The figure shows three views and two pictorial views of one solid part (mm, origin at its lowest corner). Answer the questions. Round coordinates to 2 decimals unless told otherwise and drop trailing zeros. Order: outer loops, then holes, each group sorted by start corner. A loop starts at its lowest first (then second) coordinate and runs counter-clockwise, first axis right, second up. Notation, with made-up numbers: (-18.5, 71) -> (-12.5, 71) arc R18 cw to (-12.5, 99) -> close; hole circle Ø11 at (59, 30.25). An arc over 180 degrees is marked (long way). One line per item, written item: value. Start each with the question number.
1. Section D-D (x = 7) is taken. Give the vertices of the cut face in (y, z).
2. Flat-ended cylindrical pins translate along their axes: pin 1 Ø1.5 at (y, z) = (1, 1.5) entering from -X; pin 2 Ø1.5 at (y, z) = (1, 55) entering from -X. Find the tip coordinate at first contact, or state that the pin passes through.
3. Consider line 1 (X direction, y = 0.2, z = 60); line 2 (Z direction, x = 29, y = 2.15); line 3 (X direction, y = 2.05, z = 71). Determine where each line is inside the solid, lowest interval first.
4. Section B-B (y = 2.55) is taken. Give the vertices of the cut face in (x, z), then the cut area to 3 significant figures.
5. Section A-A (z = 49.5) is taken. Give the vertices of the cut face in (x, y).
6. Section C-C (x = 21) is taken. Give the vertices of the cut face in (y, z), then the cut area to 3 significant figures.
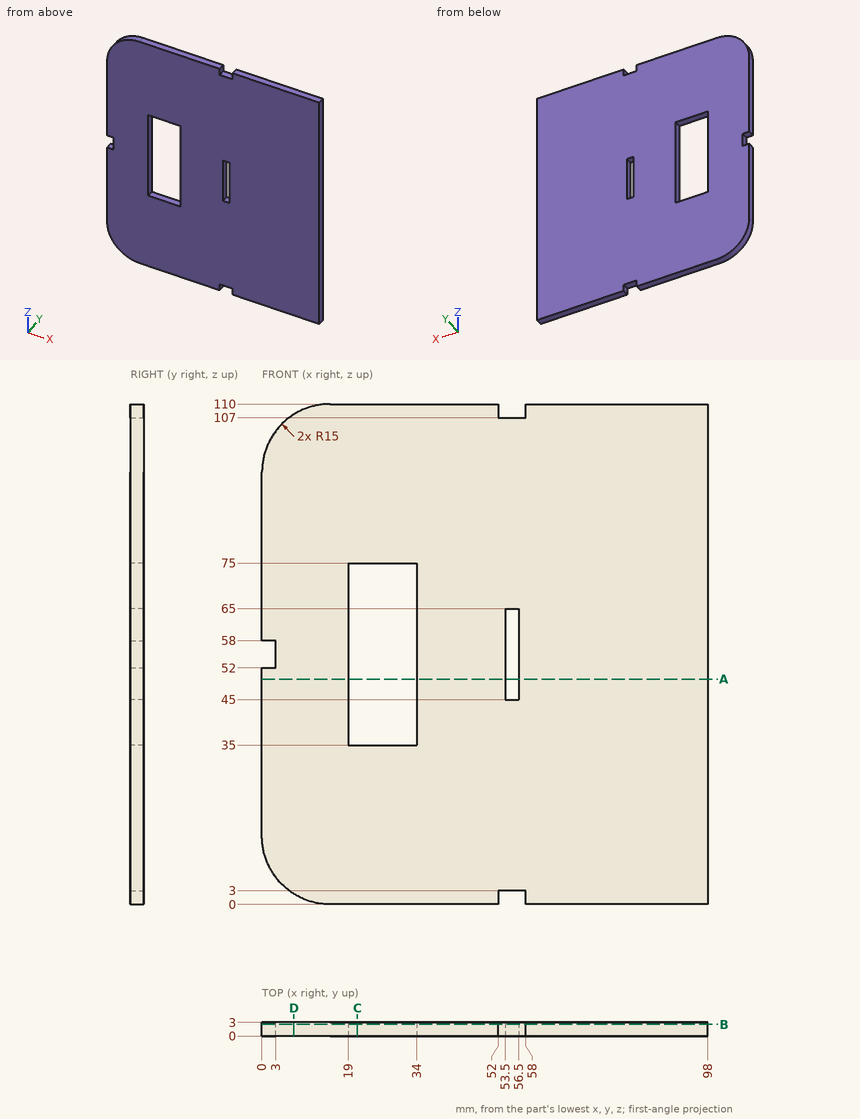
Answer:
1. outline: (0, 2.31) -> (3, 2.31) -> (3, 107.69) -> (0, 107.69) -> close
2. pin 1: x = 7.1
2. pin 2: x = 3
3. line 1: 0 to 19, 34 to 53.5, 56.5 to 98
3. line 2: 0 to 35, 75 to 110
3. line 3: 0 to 19, 34 to 98
4. outline: (0, 15) arc R15 ccw to (15, 0) -> (52, 0) -> (52, 3) -> (58, 3) -> (58, 0) -> (98, 0) -> (98, 110) -> (58, 110) -> (58, 107) -> (52, 107) -> (52, 110) -> (15, 110) arc R15 ccw to (0, 95) -> (0, 58) -> (3, 58) -> (3, 52) -> (0, 52) -> close; hole (19, 35) -> (34, 35) -> (34, 75) -> (19, 75) -> close; hole (53.5, 45) -> (56.5, 45) -> (56.5, 65) -> (53.5, 65) -> close
4. area: 9,970 mm^2
5. outline: (0, 0) -> (19, 0) -> (19, 3) -> (0, 3) -> close; (34, 0) -> (53.5, 0) -> (53.5, 3) -> (34, 3) -> close; (56.5, 0) -> (98, 0) -> (98, 3) -> (56.5, 3) -> close
6. outline: (0, 0) -> (3, 0) -> (3, 35) -> (0, 35) -> close; (0, 75) -> (3, 75) -> (3, 110) -> (0, 110) -> close
6. area: 210 mm^2
